Check sheet for the modelled part. Datum: model origin and axes. Units: mm. A direction names the side the tool comes from. Give positions to 0.01 mm unless a question says otherwise; leave off trailing zeros. Write each loop counter-clockwise with the first axis right and the second up, starting at its lowest first coordinate (ties: lowest second). Pieces come first, ordered by that corner, then holes. Notation, with made-up numbers: M 55,24.5 L 75,24.5 A16 cw 75,54.5 Z; hole C -9.75,35.25 d5. An arc over 180 degrees is marked long. Write item = value, one per line. Start each with the question number.
1) Sectioned sample at C-C, the plane z = 5.5. Record the cut outline in (x, y), then the cut area to 3 significant figures.
2) Sectioned sample at A-A, the plane x = -27.3. Record the cut outline in (y, z), then the cut area to 3 significant figures.
3) Sectioned sample at D-D, the plane x = -36.5. Record the cut outline in (y, z).
4) Sectioned sample at B-B, the plane y = 3. Record the cut outline in (x, z), then the cut area to 3 significant figures.
5) Gauge pin test, flat ends, axial feed: pin 1 (7 mm diameter, centred on x = -34, y = 3.5, fed in from -Z); pin 2 (8 mm diameter, centred on y = 17, z = -9.5, fed in from +X). Record the tip position at first contact, or that the pin passes through.
6) Set-up check for faces 5 (the face through (-29, 0, -11)), 6 (the face through (45.26, -4.26, 2.98)), 7 (the face through (-1, 22.15, 0)): record each of +Z, -Z, +X, -X, +Y, -Y from which the full face is reachable in a straight line by a thin tool's end or side.
7) Draft check along X on faces 1 (the face through (1, -22.15, 0)), 2 (the face through (-29, -20.15, -13)), 3 (the face through (-42.8, 0, 0)), 4 (the face through (-29, 20.15, -13)). Enter one of: pulls with the +X half, pulls with the -X half, needs draft (parallel to the pull), parting line crosses it, or undercut.
8) Scan lines: L1, parallel to Z at x = -27.3, y = -1; L2, parallel to X at y = -5, z = -9; L3, parallel to Z at x = -9, y = -9.5. Record each from-to range of solid material in increasing order.
Autodesk Inventor part; units mm, degrees
ref_plane "YZ Plane" through (0, 0, 0) normal (1, 0, 0) x (0, 1, 0)
ref_plane "XZ Plane" through (0, 0, 0) normal (0, 1, 0) x (-1, 0, 0)
ref_plane "XY Plane" through (0, 0, 0) normal (0, 0, 1) x (1, 0, 0)
sketch "Эскиз1" plane through (0, 0, 0) normal (0, 0, 1) x (1, 0, 0)
  line L0 (-42.8, 22.15) -> (42.8, 22.15)
  line L1 (42.8, 22.15) -> (42.8, -22.15)
  line L2 (42.8, -22.15) -> (-42.8, -22.15)
  line L3 (-42.8, -22.15) -> (-42.8, 22.15)
  line L4 (-42.8, 22.15) -> (42.8, -22.15) construction
  line L5 (42.8, 22.15) -> (-42.8, -22.15) construction
  point P0 (0, 0)
  dimension "d0" = 85.6
  dimension "d1" = 44.3
extrude "Выдавливание1" add sketch "Эскиз1" along normal mid plane 28
sketch "Эскиз2" plane through (0, 0, 14) normal (0, 0, 1) x (1, 0, 0)
  line L0 (-1.2, -2.15) -> (20.8, -2.15)
  line L1 (20.8, -2.15) -> (20.8, -22.15)
  line L2 (20.8, -22.15) -> (-1.2, -22.15)
  line L3 (-1.2, -22.15) -> (-1.2, -2.15)
  line L4 (-42.8, -22.15) -> (42.8, -22.15)
  line L5 (42.8, -22.15) -> (42.8, 22.15)
  ellipse E0 centre (9.8, -12.15) end of major axis (20.8, -12.15) minor radius 10
  point P0 (0, 0)
  point P1 (20.8, -12.15)
  point P2 (9.8, -2.15)
  point P3 (9.8, -22.15)
  point P4 (-1.2, -12.15)
  dimension "d4" = 20
  dimension "d5" = 44
  dimension "d6" = 22
extrude "Выдавливание2" add sketch "Эскиз2" along normal blind 5 contours E0
sketch "Эскиз3" plane through (42.8, -22.15, 14) normal (1, 0, 0) x (0, 0, -1)
  circle A0 centre (12, 13.5) radius 4.5
  line L0 (28, 0) -> (0, 0)
  line L1 (0, 0) -> (0, 44.3)
  point P0 (14, 22.15)
  dimension "d9" = 13.5
  dimension "d10" = 9
  dimension "d22" = 12
extrude "Выдавливание3" add sketch "Эскиз3" along normal blind 5
sketch "Эскиз4" plane through (-42.8, -22.15, -14) normal (0, -1, 0) x (1, 0, 0)
  circle A0 centre (15.5, 14) radius 7.5
  line L0 (0, 28) -> (0, 0)
  line L1 (0, 28) -> (52.6, 28)
  point P0 (42.8, 14)
  point P1 (41.6, 23)
  dimension "d13" = 15
  dimension "d14" = 15.5
  dimension "d21" = 14
extrude "Выдавливание4" cut sketch "Эскиз4" against normal through all
sketch "Эскиз5" plane through (0, 0, -14) normal (0, 0, -1) x (-1, 0, 0)
  line L0 (-42.8, -22.15) -> (42.8, -22.15)
  line L1 (42.8, -22.15) -> (42.8, 22.15)
  line L2 (42.8, 22.15) -> (-42.8, 22.15)
  line L3 (-42.8, 22.15) -> (-42.8, -22.15)
  line L4 (-40.8, 20.15) -> (40.8, 20.15)
  line L5 (40.8, 20.15) -> (40.8, -20.15)
  line L6 (40.8, -20.15) -> (-40.8, -20.15)
  line L7 (-40.8, -20.15) -> (-40.8, 20.15)
  line L8 (17.8, 20.15) -> (17.8, -20.15)
  dimension "d23" = 2
  dimension "d24" = 23
extrude "Выдавливание5" cut sketch "Эскиз5" against normal blind 3 contours L4 L5 L6 L8
properties part number "ЛЦМК0000002.00.00.00.00.05"
Data:
q1.outline = M -42.8,-22.15 L -32.4,-22.15 L -32.4,22.15 L -42.8,22.15 Z; M -22.2,-22.15 L 42.8,-22.15 L 42.8,-11.48 L 47.8,-11.48 L 47.8,-5.82 L 42.8,-5.82 L 42.8,22.15 L -22.2,22.15 Z
q1.area = 3,370 mm2
q2.outline = M -22.15,-14 L -20.15,-14 L -20.15,-11 L 20.15,-11 L 20.15,-14 L 22.15,-14 L 22.15,-7.5 L -22.15,-7.5 Z; M -22.15,7.5 L 22.15,7.5 L 22.15,14 L -22.15,14 Z
q2.area = 455 mm2
q3.outline = M -22.15,-14 L -20.15,-14 L -20.15,-11 L 20.15,-11 L 20.15,-14 L 22.15,-14 L 22.15,14 L -22.15,14 Z
q4.outline = M -42.8,-14 L -40.8,-14 L -40.8,-11 L -17.8,-11 L -17.8,-14 L 42.8,-14 L 42.8,14 L -42.8,14 Z; hole C -27.3,0 d15
q4.area = 2,150 mm2
q5.pin_1 = -11
q5.pin_2 = 42.8
q6.face_5 = -Z
q6.face_6 = +X
q6.face_7 = +Z, -Z, +X, -X, +Y
q7.face_1 = needs draft
q7.face_2 = undercut
q7.face_3 = pulls with the -X half
q7.face_4 = undercut
q8.L1 = -11 to -7.5, 7.5 to 14
q8.L2 = -42.8 to 42.8
q8.L3 = -14 to 14
